```python
from build123d import *

# Parameters (mm, degrees)
SKETCH3_R           = 6.35
SKETCH3_R_2         = 1.25
BOSS_EXTRUDE4_DEPTH = 3.175


with BuildPart() as part:
    # Sketch3 → Boss-Extrude4 (new body, symmetric)
    with BuildSketch(Plane(origin=(0, 0, 0), x_dir=(1, 0, 0), z_dir=(0, 1, 0))):
        with BuildLine():
            Line((-25.4, 0), (-25.4, -25.4))
            Line((-25.4, -25.4), (0, -25.4))
            Line((0, -25.4), (25.4, -25.4))
            Line((25.4, -25.4), (25.4, 0))
            ThreePointArc((25.4, 0), (0, 25.4), (-25.4, 0))
        make_face()
        with Locations((1e-09, 7)):
            Circle(SKETCH3_R, mode=Mode.SUBTRACT)
        with Locations((7.75, 13.423393759)):
            Circle(SKETCH3_R_2, mode=Mode.SUBTRACT)
        with Locations((-7.75, 13.423393759)):
            Circle(SKETCH3_R_2, mode=Mode.SUBTRACT)
        with Locations((-7.75, -13.423393759)):
            Circle(SKETCH3_R_2, mode=Mode.SUBTRACT)
        with Locations((7.75, -13.423393759)):
            Circle(SKETCH3_R_2, mode=Mode.SUBTRACT)
    extrude(amount=BOSS_EXTRUDE4_DEPTH, both=True)


solid = part.part
```
Verification items for the finished model (mm, model axes). Give positions to 0.01 mm unless a question says otherwise; leave off trailing zeros. Loops run counter-clockwise (first coordinate to the right, second up) from the corner with the lowest first, then second, coordinate; pieces in that order, holes last.
1. Mould release check, pull along X, two halves, no side actions. Record for faces 1 (the cylindrical face through (-1.38, -0.04, -0.8)), 2 (the flat face through (-25.4, 0, 13)), 3 (the flat face through (0, 0, 25.4)): released by +X, released by -X, zero draft, split by the parting line, or undercut.
2. Section check A-A, the plane x = 0. Enter the section's corners in (y, z) (3 decimals), then the cut area to 3 significant figures.
3. Go/stop test with a flat-tipped pin: pin 1 Ø3 at (y, z) = (1.5, -7) entering from +X. Record where the tip stops, or that it passes through.
4. Thickness scan on line 1 (Z direction, x = -7.75, y = 1.25); line 2 (X direction, y = 1, z = -14); line 3 (Z direction, x = 0, y = -1.25). Record the ranges inside material, lowest first.
5. Section check C-C, the plane x = 7.75. Enter the section's corners in (y, z) (3 decimals), then the cut area to 3 significant figures.
6. Section check D-D, the plane y = 2. Enter the section's corners in (x, z).
7. Section check B-B, the plane z = -1.5. Enter the section's corners in (x, y) (3 decimals).
Geometry says:
1. face 1: undercut
1. face 2: released by -X
1. face 3: zero draft
2. outline: (-3.175, -25.4) - (3.175, -25.4) - (3.175, -13.35) - (-3.175, -13.35) - close; (-3.175, -0.65) - (3.175, -0.65) - (3.175, 25.4) - (-3.175, 25.4) - close
2. area: 242 mm2
3. pin 1: stops at x = 24.8
4. line 1: z = -24.19 to -14.67, -12.17 to 12.17, 14.67 to 25.4
4. line 2: x = -21.19 to -8.86, -6.64 to 6.64, 8.86 to 21.19
4. line 3: z = -25.4 to -13.35, -0.65 to 25.4
5. outline: (-3.175, -24.189) - (3.175, -24.189) - (3.175, -14.673) - (-3.175, -14.673) - close; (-3.175, -12.173) - (3.175, -12.173) - (3.175, 12.173) - (-3.175, 12.173) - close; (-3.175, 14.673) - (3.175, 14.673) - (3.175, 25.4) - (-3.175, 25.4) - close
5. area: 283 mm2
6. outline: (-25.4, 0) arc R25.4 ccw to (25.4, 0) - (25.4, 25.4) - (-25.4, 25.4) - close; hole circle Ø2.5 at (-7.75, -13.42); hole circle Ø2.5 at (-7.75, 13.42); hole circle Ø12.7 at (0, -7); hole circle Ø2.5 at (7.75, -13.42); hole circle Ø2.5 at (7.75, 13.42)
7. outline: (-25.356, -3.175) - (-3.174, -3.175) - (-3.174, 3.175) - (-25.356, 3.175) - close; (3.174, -3.175) - (25.356, -3.175) - (25.356, 3.175) - (3.174, 3.175) - close
